Autodesk Inventor part; units mm, degrees
ref_plane "YZ Plane" through (0, 0, 0) normal (1, 0, 0) x (0, 1, 0)
ref_plane "XZ Plane" through (0, 0, 0) normal (0, 1, 0) x (-1, 0, 0)
ref_plane "XY Plane" through (0, 0, 0) normal (0, 0, 1) x (1, 0, 0)
sketch "스케치1" plane through (0, 0, 0) normal (0, 0, 1) x (1, 0, 0)
  line L0 (-24.8745, -28.5) -> (-24.8745, -22.5)
  line L1 (-24.8745, -22.5) -> (-24.6915, -22.5)
  line L2 (4.8745, -22.5) -> (4.8745, -28.5)
  line L3 (30, -28.5) -> (4.8745, -28.5)
  line L4 (30, 27.5) -> (30, -28.5)
  line L5 (30, 27.5) -> (4.8745, 27.5)
  line L6 (4.8745, 27.5) -> (4.8745, 21.5)
  line L7 (-24.6915, 21.5) -> (-24.8745, 21.5)
  line L8 (-24.8745, 21.5) -> (-24.8745, 27.5)
  line L9 (17, -7.5) -> (25, -7.5)
  line L10 (25, -7.5) -> (25, 6.5)
  line L11 (25, 6.5) -> (17, 6.5)
  line L12 (17, 6.5) -> (17, -7.5)
  arc A0 (19.7598, -5.3438) -> (22.2402, -5.3438) centre (21, -5.5) ccw
  arc A1 (22.2402, 4.3437) -> (19.7598, 4.3437) centre (21, 4.5) ccw
  circle A2 centre (21, -5.5) radius 0.9
  circle A3 centre (21, 4.5) radius 0.9
  arc A4 (19.7598, 4.3437) -> (19.7598, -5.3438) centre (21, -0.5) ccw
  arc A5 (22.2402, -5.3438) -> (22.2402, 4.3437) centre (21, -0.5) ccw
  circle A6 centre (21, -5.5) radius 0.9
  circle A7 centre (21, 4.5) radius 0.9
  line L13 (-21.6915, -12.5) -> (-21.6915, 11.5)
  line L14 (4, 11.5) -> (4, -12.5)
  line L15 (-24.8745, 27.5) -> (-33, 27.5)
  line L16 (-33, -28.5) -> (-33, 27.5)
  line L17 (-24.8745, -28.5) -> (-33, -28.5)
  line L18 (7, -22.5) -> (4.8745, -22.5)
  line L19 (4.8745, 21.5) -> (7, 21.5)
  line L20 (7, 21.5) -> (7, 20)
  line L21 (7, 20) -> (-24.6915, 20)
  line L22 (-24.6915, 20) -> (-24.6915, 21.5)
  line L23 (-24.6915, -22.5) -> (-24.6915, -21)
  line L24 (-24.6915, -21) -> (7, -21)
  line L25 (7, -21) -> (7, -22.5)
  line L26 (4, -12.5) -> (-21.6915, -12.5)
  line L27 (-21.6915, 11.5) -> (4, 11.5)
  point P0 (0, 0)
  dimension "d0" = 8
  dimension "d1" = 5
  dimension "d2" = 14
  dimension "d3" = 56
  dimension "d4" = 21
  dimension "d5" = 2.5
  dimension "d6" = 2.5
  dimension "d7" = 10
  dimension "d8" = 2
  dimension "d9" = 4
  dimension "d10" = 4
  dimension "d11" = 1.8
  dimension "d12" = 1.8
  dimension "d13" = 21
  dimension "d14" = 2
extrude "돌출1" add sketch "스케치1" along normal blind 1 contours A4 L12 | L12 A4 A1 A5 L10 A0 | L10 A5
sketch "스케치2" plane through (0, 0, 1) normal (0, 0, 1) x (1, 0, 0)
  arc A0 (19.7598, 4.3437) -> (19.7598, -5.3438) centre (21, -0.5) ccw
  arc A1 (22.2402, 4.3437) -> (19.7598, 4.3437) centre (21, 4.5) ccw
  arc A2 (22.2402, -5.3438) -> (22.2402, 4.3437) centre (21, -0.5) ccw
  arc A3 (19.7598, -5.3438) -> (22.2402, -5.3438) centre (21, -5.5) ccw
  arc A4 (19.2637, 4.7187) -> (19.2637, -5.7188) centre (21, -0.5) ccw
  arc A5 (22.7363, 4.7187) -> (19.2637, 4.7187) centre (21, 4.5) ccw
  arc A6 (22.7363, -5.7188) -> (22.7363, 4.7187) centre (21, -0.5) ccw
  arc A7 (19.2637, -5.7188) -> (22.7363, -5.7188) centre (21, -5.5) ccw
  point P0 (0, 0)
  dimension "d17" = 0.5
extrude "돌출2" add sketch "스케치2" against normal blind 1
sketch "스케치3" plane through (0, 0, 1) normal (0, 0, 1) x (1, 0, 0)
  arc A0 (19.2637, 4.7187) -> (19.2637, -5.7188) centre (21, -0.5) ccw
  arc A1 (19.2637, -5.7188) -> (22.7363, -5.7188) centre (21, -5.5) ccw
  arc A2 (22.7363, -5.7188) -> (22.7363, 4.7187) centre (21, -0.5) ccw
  arc A3 (22.7363, 4.7187) -> (19.2637, 4.7187) centre (21, 4.5) ccw
  circle A4 centre (21, 4.5) radius 0.9
  circle A5 centre (21, -5.5) radius 0.9
  point P0 (0, 0)
extrude "돌출3" add sketch "스케치3" along normal blind 1
sketch "스케치4" plane through (0, 0, 2) normal (0, 0, 1) x (1, 0, 0)
  circle A0 centre (21, -5.5) radius 0.9
  circle A1 centre (21, 4.5) radius 0.9
  arc A2 (19.2637, 4.7187) -> (19.2637, -5.7188) centre (21, -0.5) ccw
  arc A3 (19.2637, -5.7188) -> (22.7363, -5.7188) centre (21, -5.5) ccw
  arc A4 (22.7363, -5.7188) -> (22.7363, 4.7187) centre (21, -0.5) ccw
  arc A5 (22.7363, 4.7187) -> (19.2637, 4.7187) centre (21, 4.5) ccw
  circle A6 centre (21, -0.5) radius 3
  point P0 (0, 0)
  dimension "d22" = 6
extrude "돌출4" add sketch "스케치4" along normal blind 4 contours A6
fillet "모깎기1" radius 2 1 edges at (18, -0.5, 6)
properties part number "candynamix_mini_ballcaster"
Verification items for the finished model (mm, model axes). A direction names the side the tool comes from. Give positions to 0.01 mm unless a question says otherwise; leave off trailing zeros. Order: outer loops, then holes, each group sorted by start corner. A loop starts at its lowest first (then second) coordinate and runs counter-clockwise, first axis right, second up. Notation, with made-up numbers: (25.25, -10) -> (82.25, -10) arc R7 ccw to (82.25, 1) -> close; hole circle Ø11 at (45.25, -40). An arc over 180 degrees is marked (long way). One line per item, written item: value.
(1) Sectioned sample at D-D on x = 17.25. Record the cut outline in (y, z).
Final values:
outline: (-4.52, 0) -> (3.52, 0) -> (3.52, 2) -> (-4.52, 2) -> close
(2) Sectioned sample at C-C on z = 2.5. Record the cut outline in (x, y).
Final values:
outline: circle Ø6 at (21, -0.5)
(3) Sectioned sample at B-B on x = 21. Count the separate pieces of the cut face and the enclosed holes in it, then the cut area to 3 significant figures.
Final values:
separate pieces: 3
enclosed holes: 0
area: 42.1 mm^2
(4) Scan lines: line 1 along Y through (x, z) = (21, 0.6); line 2 along Z through (x, y) = (18.5, 4); line 3 along X through (y, z) = (-1.5, 2.25). Record each from-to range of solid material in increasing order. Write a range as [from, to].
Final values:
line 1: [-7.25, -6.4], [-4.6, 3.6], [5.4, 6.25]
line 2: [0, 2]
line 3: [18.17, 23.83]
(5) Draft check along X on faces 3 (the face through (26.5, -0.4, 1)), 4 (the face through (21.415, 5.298, 0.986)), 5 (the face through (18, -0.6, 3)), 6 (the face through (21.415, -4.702, 0.986)). Enter one of: pulls with the +X half, pulls with the -X half, needs draft (parallel to the pull), parting line crosses it, or undercut.
Final values:
face 3: pulls with the +X half
face 4: undercut
face 5: parting line crosses it
face 6: undercut
(6) Tool access check on faces 1 (the face through (21, 3, 2)), 2 (the face through (21.04, -7.25, 0.99)). Record the directions out of +Z, -Z, +X, -X, +Y, -Y that give a thin tool (end or side, any length) a straight path to the whole face; none if there is none.
Final values:
face 1: +Z
face 2: +Z, -Z, -Y
(7) Sectioned sample at A-A on y = -5.5. Record the cut outline in (x, z).
Final values:
outline: (18.71, 0) -> (20.1, 0) -> (20.1, 2) -> (18.71, 2) -> close; (21.9, 0) -> (23.29, 0) -> (23.29, 2) -> (21.9, 2) -> close
(8) Gauge pin test, flat ends, axial feed: pin 1 (1 mm diameter, centred on x = 23.5, z = 5, fed in from +Y); pin 2 (1.1 mm diameter, centred on x = 21, y = 4.5, fed in from +Z); pin 3 (1.5 mm diameter, centred on y = 4, z = 1.5, fed in from +X). Record the tip position at first contact, or that the pin passes through.
Final values:
pin 1: y = 1.47
pin 2: through
pin 3: x = 25.02
